The model under review builds one solid part; all positions refer to its coordinate system, in mm. Face numbers are marked on the shaded views. A direction names the side the tool comes from. Give positions to 0.01 mm unless a question says otherwise; leave off trailing zeros. Order: outer loops, then holes, each group sorted by start corner. A loop starts at its lowest first (then second) coordinate and runs counter-clockwise, first axis right, second up.
```python
from build123d import *

# Parameters (mm, degrees)
SKETCH1_R            = 2.5
BOSS_EXTRUDE1_DEPTH  = 29
SKETCH2_R            = 9.5
CUT_EXTRUDE1_DEPTH   = 30
SKETCH2_6_R          = 9.5
SKETCH2_6_R_2        = 2.5
SKETCH2_6_R_3        = 1.5
CUT_EXTRUDE2_DEPTH   = 1
SKETCH6_R            = 2.5
SKETCH6_R_2          = 9.5
CUT_EXTRUDE3_DEPTH   = 29
SKETCH27_R           = 2
CUT_EXTRUDE7_DEPTH   = 65
BOSS_EXTRUDE2_DEPTH  = 10
CUT_EXTRUDE4_DEPTH   = 7
BOSS_EXTRUDE3_DEPTH  = 1
SKETCH13_R           = 10.5
BOSS_EXTRUDE4_DEPTH  = 1.5
BOSS_EXTRUDE4_TAPER  = 36
SKETCH14_R           = 3.5
BOSS_EXTRUDE5_DEPTH  = 8
BOSS_EXTRUDE6_DEPTH  = 2
BOSS_EXTRUDE6_TAPER  = 29
SKETCH18_R           = 4.491355914
BOSS_EXTRUDE7_DEPTH  = 9
BOSS_EXTRUDE8_DEPTH  = 2
SKETCH20_R           = 4
SKETCH20_R_2         = 2.5
BOSS_EXTRUDE9_DEPTH  = 1
BOSS_EXTRUDE10_DEPTH = 6
SKETCH25_R           = 0.5
CUT_EXTRUDE5_DEPTH   = 9
SKETCH26_R           = 0.75
CUT_EXTRUDE6_DEPTH   = 9


with BuildPart() as part:
    # Sketch1 → Boss-Extrude1 (new body)
    with BuildSketch(Plane.XY):
        with BuildLine():
            Line((-14.028828829, 0), (19.971171171, 0))
            Line((19.971171171, 0), (23.476315099, 4.036089643))
            Line((23.476315099, 4.036089643), (22.286560603, 5.069332489))
            Line((22.286560603, 5.069332489), (25.250471061, 10.500003392))
            ThreePointArc((25.250471061, 10.500003392), (30.244646337, 15.502911939), (25.244647185, 20.5))
            Line((25.244647185, 20.5), (25.244647185, 28.5))
            Line((25.244647185, 28.5), (-3.755352815, 28.5))
            Line((-3.755352815, 28.5), (-7.213070041, 19))
            Line((-7.213070041, 19), (-14.028828829, 19))
            Line((-14.028828829, 19), (-14.028828829, 0))
        make_face()
        with Locations((25.244647185, 15.5)):
            Circle(SKETCH1_R, mode=Mode.SUBTRACT)
    extrude(amount=BOSS_EXTRUDE1_DEPTH)

    # Sketch2 → Cut-Extrude1 (cut, through all)
    with BuildSketch(Plane.XY.offset(29)):
        with Locations((10.744647185, 15.5)):
            Circle(SKETCH2_R)
    extrude(amount=-CUT_EXTRUDE1_DEPTH, mode=Mode.SUBTRACT)

    # Sketch2_6 → Cut-Extrude2 (cut)
    with BuildSketch(Plane.XY.offset(29)):
        with Locations((10.744647185, 15.5)):
            Circle(SKETCH2_6_R)
        with Locations((-3.755352815, 15.5)):
            Circle(SKETCH2_6_R_2)
        with Locations((21.22529921, 24.036089643)):
            Circle(SKETCH2_6_R_3)
        with Locations((-0.698224059, 24.036089643)):
            Circle(SKETCH2_6_R_3)
        with Locations((19.301775941, 4.036089643)):
            Circle(SKETCH2_6_R_3)
        with Locations((-0.698224059, 4.036089643)):
            Circle(SKETCH2_6_R_3)
    extrude(amount=-CUT_EXTRUDE2_DEPTH, mode=Mode.SUBTRACT)

    # Sketch6 → Cut-Extrude3 (cut, through all)
    with BuildSketch(Plane.XY.offset(28)):
        with Locations((-3.755352815, 15.5)):
            Circle(SKETCH6_R)
        with Locations((25.244647185, 15.5)):
            Circle(SKETCH6_R)
        with Locations((10.744647185, 15.5)):
            Circle(SKETCH6_R_2)
    extrude(amount=-CUT_EXTRUDE3_DEPTH, mode=Mode.SUBTRACT)

    # Sketch27 → Cut-Extrude7 (cut)
    with BuildSketch(Plane(origin=(15.039946678, -8.208388255, 0), x_dir=(0, 0, -1), z_dir=(0.877778246, -0.479067167, 0))):
        with Locations((-26, 18.313346199)):
            Circle(SKETCH27_R)
        with Locations((-4, 18.313346199)):
            Circle(SKETCH27_R)
    extrude(amount=-CUT_EXTRUDE7_DEPTH, mode=Mode.SUBTRACT)

    # Sketch10 → Boss-Extrude2 (add)
    with BuildSketch(Plane.ZY.offset(14.028828829)):
        with BuildLine():
            Line((11, 0), (25, 0))
            Line((25, 0), (25, 2.052918349))
            ThreePointArc((25, 2.052918349), (25.674542678, 7.876031451), (20.714252914, 11))
            Line((20.714252914, 11), (15, 11))
            ThreePointArc((15, 11), (9.949651265, 7.678067412), (11, 1.725082782))
            Line((11, 1.725082782), (11, 0))
        make_face()
        with BuildLine():
            ThreePointArc((17.857126457, 3.478409436), (24.214252914, 5.5), (17.857126457, 7.521590564))
            ThreePointArc((17.857126457, 7.521590564), (11.5, 5.5), (17.857126457, 3.478409436))
        make_face(mode=Mode.SUBTRACT)
    extrude(amount=BOSS_EXTRUDE2_DEPTH)

    # Sketch11 → Cut-Extrude4 (cut)
    with BuildSketch(Plane.ZY.offset(14.028828829)):
        with BuildLine():
            Line((9.5, 5.5), (9.5, 19))
            Line((9.5, 19), (9.5, 20))
            Line((9.5, 20), (20.714252914, 20))
            Line((20.714252914, 20), (20.714252914, 19))
            Line((20.714252914, 19), (20.714252914, 11))
            Line((20.714252914, 11), (15, 11))
            ThreePointArc((15, 11), (11.110912703, 9.389087297), (9.5, 5.5))
        make_face()
    extrude(amount=-CUT_EXTRUDE4_DEPTH, mode=Mode.SUBTRACT)

    # Sketch12 → Boss-Extrude3 (add)
    with BuildSketch(Plane.XZ):
        with BuildLine():
            Line((-5.928828829, 27.5), (17.071171171, 27.5))
            ThreePointArc((17.071171171, 27.5), (18.485384734, 26.914213562), (19.071171171, 25.5))
            Line((19.071171171, 25.5), (19.071171171, 3.5))
            ThreePointArc((19.071171171, 3.5), (18.485384734, 2.085786438), (17.071171171, 1.5))
            Line((17.071171171, 1.5), (-5.928828829, 1.5))
            ThreePointArc((-5.928828829, 1.5), (-7.343042391, 2.085786438), (-7.928828829, 3.5))
            Line((-7.928828829, 3.5), (-7.928828829, 25.5))
            ThreePointArc((-7.928828829, 25.5), (-7.343042391, 26.914213562), (-5.928828829, 27.5))
        make_face()
    extrude(amount=BOSS_EXTRUDE3_DEPTH)

    # Sketch13 → Boss-Extrude4 (add)
    with BuildSketch(Plane.XZ.offset(1)):
        with Locations((5.571171171, 14.5)):
            Circle(SKETCH13_R)
    extrude(amount=BOSS_EXTRUDE4_DEPTH, taper=BOSS_EXTRUDE4_TAPER)

    # Sketch14 → Boss-Extrude5 (add)
    with BuildSketch(Plane(origin=(25.244647185, 0, 0), x_dir=(0, 0, -1), z_dir=(1, 0, 0))):
        with Locations((-6, 24.5)):
            Circle(SKETCH14_R)
    extrude(amount=BOSS_EXTRUDE5_DEPTH)

    # Sketch16 → Revolve1 (revolve)
    with BuildSketch(Plane.ZX.offset(24.5)):
        Polygon((8.87886056, 33.244647185), (12, 32.59776031), (12, 33.244647185), (14, 32.59776031), (14, 32.871461105), (15.5, 32.386295949), (15.5, 31.707729006), (9.5, 31.707729006), (8.87886056, 31.707729006), align=None)
    revolve(axis=Axis((31.707729006, 24.5, 15.5), (0, 0, -1)))

    # Sketch17 → Boss-Extrude6 (add)
    with BuildSketch(Plane(origin=(0, 28.5, 0), x_dir=(1, 0, 0), z_dir=(0, 1, 0))):
        with BuildLine():
            Line((23.244647185, 0), (-1.755352815, 0))
            ThreePointArc((-1.755352815, 0), (-3.169566378, -0.585786438), (-3.755352815, -2))
            Line((-3.755352815, -2), (-3.755352815, -27))
            ThreePointArc((-3.755352815, -27), (-3.169566378, -28.414213562), (-1.755352815, -29))
            Line((-1.755352815, -29), (23.244647185, -29))
            ThreePointArc((23.244647185, -29), (24.658860747, -28.414213562), (25.244647185, -27))
            Line((25.244647185, -27), (25.244647185, -2))
            ThreePointArc((25.244647185, -2), (24.658860747, -0.585786438), (23.244647185, 0))
        make_face()
    extrude(amount=BOSS_EXTRUDE6_DEPTH, taper=BOSS_EXTRUDE6_TAPER)

    # Sketch18 → Boss-Extrude7 (add)
    with BuildSketch(Plane(origin=(0, 30.5, 0), x_dir=(1, 0, 0), z_dir=(0, 1, 0))):
        with Locations((7.267412162, -8.971106597)):
            Circle(SKETCH18_R)
    extrude(amount=BOSS_EXTRUDE7_DEPTH)

    # Sketch19 → Boss-Extrude8 (add)
    with BuildSketch(Plane(origin=(0, 30.5, 0), x_dir=(1, 0, 0), z_dir=(0, 1, 0))):
        with BuildLine():
            Line((-10.646734712, -25.108618103), (-14.646734712, -23.108618103))
            Line((-14.646734712, -23.108618103), (-14.646734712, -13.108618103))
            Line((-14.646734712, -13.108618103), (-8.646734712, -13.108618103))
            Line((-8.646734712, -13.108618103), (-8.646734712, -23.108618103))
            Line((-8.646734712, -23.108618103), (-2.646734712, -23.108618103))
            Line((-2.646734712, -23.108618103), (-2.646734712, -17.108618103))
            Line((-2.646734712, -17.108618103), (4.687209994, -17.108618103))
            ThreePointArc((4.687209994, -17.108618103), (8.520237641, -21.275590456), (4.353265288, -25.108618103))
            Line((4.353265288, -25.108618103), (-2.646734712, -25.108618103))
            Line((-2.646734712, -25.108618103), (-10.646734712, -25.108618103))
        make_face()
    extrude(amount=BOSS_EXTRUDE8_DEPTH)

    # Sketch20 → Boss-Extrude9 (add)
    with BuildSketch(Plane(origin=(0, 32.5, 0), x_dir=(1, 0, 0), z_dir=(0, 1, 0))):
        with Locations((4.520237641, -21.108618103)):
            Circle(SKETCH20_R)
        with Locations((4.520237641, -21.108618103)):
            Circle(SKETCH20_R_2, mode=Mode.SUBTRACT)
    extrude(amount=BOSS_EXTRUDE9_DEPTH)

    # Sketch22 → Revolve2 (revolve)
    with BuildSketch(Plane(origin=(0, 0, 8.971106597), x_dir=(-1, 0, 0), z_dir=(0, 0, -1))):
        Polygon((-17.615312055, 37.490470155), (-10.736326453, 37.490470155), (-10.736326453, 39.5), (-13.578550719, 38.558914033), (-13.578550719, 39.5), (-15.893217754, 38.733592967), (-15.893217754, 39.116796484), (-17.615312055, 38.558914033), align=None)
    revolve(axis=Axis((17.615312055, 37.490470155, 8.971106597), (-1, 0, 0)))

    # Sketch24 → Boss-Extrude10 (add)
    with BuildSketch(Plane(origin=(-8.646734712, 0, 0), x_dir=(0, 0, -1), z_dir=(1, 0, 0))):
        Polygon((-21.108618103, 32.5), (-18.108618103, 30.5), (-23.108618103, 30.5), (-23.108618103, 32.5), align=None)
    extrude(amount=BOSS_EXTRUDE10_DEPTH)

    # Sketch25 → Cut-Extrude5 (cut)
    with BuildSketch(Plane.XY.offset(15.5)):
        with Locations((31.707729006, 24.5)):
            Circle(SKETCH25_R)
    extrude(amount=-CUT_EXTRUDE5_DEPTH, mode=Mode.SUBTRACT)

    # Sketch26 → Cut-Extrude6 (cut)
    with BuildSketch(Plane(origin=(17.615312055, 0, 0), x_dir=(0, 0, -1), z_dir=(1, 0, 0))):
        with Locations((-8.971106597, 37.490470155)):
            Circle(SKETCH26_R)
    extrude(amount=-CUT_EXTRUDE6_DEPTH, mode=Mode.SUBTRACT)


solid = part.part
```
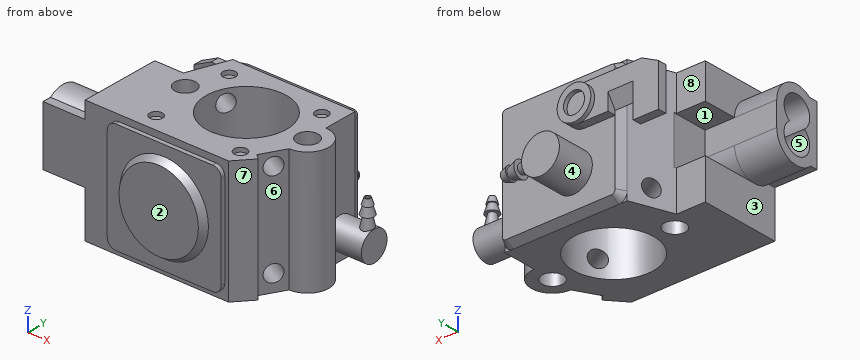
1. Take a section at A-A (y = 15.5). Write out the cut boundary in (x, z).
2. To check wall thickness, follow line 1 (Z direction, x = -18, y = 5.5); line 2 (Z direction, x = -19, y = 3); line 3 (Y direction, x = 13.5, z = 18.25). State the ranges of each line that lie inside material, in increasing order.
3. For the marked faces 4, 5, 6, 7 and 8, list the 3-axis set-ups (+Z, -Z, +X, -X, +Y, -Y) from which the entire face can be reached by the end or side of a thin tool; tool diameter is ignored.
4. Insertion check: pin 1 (1 mm diameter, centred on y = 9.5, z = 24, fed in from +X); pin 2 (1 mm diameter, centred on x = -5.5, y = 32, fed in from +Z); pin 3 (3.5 mm diameter, centred on x = -10, z = 24.5, fed in from +Y). Each pin has a flat end and moves straight along its axis. Give the tip position at first contact, or say it passes through.
5. Draft analysis for pull direction Y (two halves, no side actions). For the marked faces 1, 2 and 3, state which applies: pulls with the +Y half, pulls with the -Y half, needs draft (parallel to the pull), parting line crosses it, or undercut.
Answer:
1. outline: (-14.03, 0) - (-6.26, 0) - (-6.26, 29) - (-14.03, 29) - (-14.03, 20.71) - (-7.03, 20.71) - (-7.03, 9.5) - (-14.03, 9.5) - close; (-1.26, 0) - (1.24, 0) - (1.24, 29) - (-1.26, 29) - close; (20.24, 0) - (22.74, 0) - (22.74, 29) - (20.24, 29) - close; (27.74, 0) - (30.24, 0) - (30.24, 29) - (27.74, 29) - close
2. line 1: z = 9.5 to 11.5, 24.21 to 26.21
2. line 2: z = 10.1 to 12.55, 17.45 to 18.26, 23.16 to 25.61
2. line 3: y = -2.5 to 6.41, 24.59 to 30.5
3. face 4: none
3. face 5: -X
3. face 6: +Z, -Z, +X
3. face 7: +Z, -Z, +X, -Y
3. face 8: +Z, -Z, -X
4. pin 1: stops at x = 24.98
4. pin 2: stops at z = 25.11
4. pin 3: stops at y = 32.5
5. face 1: undercut
5. face 2: pulls with the -Y half
5. face 3: needs draft
